CAD build for the part. Positions are in the model's coordinates, mm. A direction names the side the tool comes from. Coordinates: 2 decimals unless noted, no trailing zeros. Write each loop counter-clockwise with the first axis right and the second up, starting at its lowest first coordinate (ties: lowest second). Pieces come first, ordered by that corner, then holes. Notation, with made-up numbers: (79.25, 60.5) - (89.25, 60.5) arc R18 ccw to (89.25, 90.5) - close; hole circle Ø8 at (32, -17.75). An arc over 180 degrees is marked (long way). Answer in a Markdown table with one row per item. Add a question column.
Q1. 3-axis set-ups, long thin cutter, end or side, ignore diameter. For faces 1 (the flat face through (0, 518, 372)), 2 (the flat face through (-25, 50, 321)), 3 (the flat face through (-50, 525, 321)): which of +Z, -Z, +X, -X, +Y, -Y reach the whole face in a straight line?
Q2. Band-saw the part on B-B (y = 481). List the corners of the cut face in (x, z).
Q3. Drill centre lines: line 1 along Z through (x, y) = (-387, 292); line 2 along Y through (x, z) = (-505.5, 617.5); line 3 along Y through (x, z) = (-517.5, 272.5). Where is each one in solid material? Low to high. Write a range as from..to.
Q4. Band-saw the part on C-C (x = -184). List the corners of the cut face in (y, z).
Q5. Band-saw the part on A-A (z = 113). List the corners of the cut face in (x, y).
Q6. Two-plate mould, pull along Y, no slides. Class faces 4 (the flat face through (-516, 550, 320)), 5 (the flat face through (-279, 279, 600)), 6 (the flat face through (-50, 25, 321)): +Y half, -Y half, draft (parallel to the pull), parting line (faces both ways), or undercut.
Q7. Band-saw the part on D-D (x = -510). List the corners of the cut face in (y, z).
Q8. Pin check, flat tips, straight feed: pin 1 (25 mm diameter, centred on y = 17.5, z = 460.5, fed in from +X); pin 2 (25 mm diameter, centred on y = -38.5, z = 151.5, fed in from -X); pin 3 (1.4 mm diameter, centred on x = 1, z = 153.5, fed in from +Y). Stop position of each tip, or through.
```python
from build123d import *

# Parameters (mm, degrees)
F0_W     = 550
F0_H     = 550
F1_DEPTH = 50
F2_W     = 50
F2_H     = 50
F3_DEPTH = 550
F4_W     = 50
F4_H     = 50
F5_DEPTH = 50
F6_W     = 82.6920196414
F6_H     = 273.0440795422
F6_W_2   = 143.6941742897
F6_H_2   = 223.0440795422
F7_DEPTH = 1.8


with BuildPart() as f1:
    # F0 (on Top) → F1 (new body)
    with BuildSketch(Plane.XY):
        with Locations((-275, 275)):
            Rectangle(F0_W, F0_H)
    extrude(amount=F1_DEPTH)

    # F2 (on face) → F3 (join)
    with BuildSketch(Plane.XY.offset(50)):
        with Locations((-525, 525)):
            Rectangle(F2_W, F2_H)
        with Locations((-525, 25)):
            Rectangle(F2_W, F2_H)
        with Locations((-25, 25)):
            Rectangle(F2_W, F2_H)
        with Locations((-25, 525)):
            Rectangle(F2_W, F2_H)
    extrude(amount=F3_DEPTH)

    # F4 (on face) → F5 (join)
    with BuildSketch(Plane.XY.offset(600)):
        with Locations((-525, 525)):
            Rectangle(F4_W, F4_H)
        Polygon((0, 550), (-500, 550), (-500, 500), (-550, 500), (-550, 0), (0, 0), align=None)
    extrude(amount=F5_DEPTH)

    # F6 (on face) → F7 (join)
    with BuildSketch(Plane.YZ):
        with Locations((-41.3460098207, 136.5220397711)):
            Rectangle(F6_W, F6_H)
        Polygon((0, 0), (193.6941742897, 0), (193.6941742897, 50), (50, 50), (50, 273.0440795422), (0, 273.0440795422), align=None)
        with Locations((121.8470871449, 161.5220397711)):
            Rectangle(F6_W_2, F6_H_2)
    extrude(amount=F7_DEPTH)


solid = f1.part
```
Checked values:
| question | item | result |
|---|---|---|
| 1 | face 1 | +Z, +X, +Y |
| 1 | face 2 | -X |
| 1 | face 3 | +Y, -Y |
| 2 | outline | (-550, 0) - (0, 0) - (0, 50) - (-550, 50) - close; (-550, 600) - (0, 600) - (0, 650) - (-550, 650) - close |
| 3 | line 1 | z = 0..50, 600..650 |
| 3 | line 2 | y = 0..550 |
| 3 | line 3 | y = 0..50, 500..550 |
| 4 | outline | (0, 0) - (550, 0) - (550, 50) - (0, 50) - close; (0, 600) - (550, 600) - (550, 650) - (0, 650) - close |
| 5 | outline | (-550, 0) - (-500, 0) - (-500, 50) - (-550, 50) - close; (-550, 500) - (-500, 500) - (-500, 550) - (-550, 550) - close; (-50, 0) - (0, 0) - (0, -82.69) - (1.8, -82.69) - (1.8, 193.69) - (0, 193.69) - (0, 50) - (-50, 50) - close; (-50, 500) - (0, 500) - (0, 550) - (-50, 550) - close |
| 6 | face 4 | +Y half |
| 6 | face 5 | undercut |
| 6 | face 6 | draft |
| 7 | outline | (0, 0) - (550, 0) - (550, 650) - (0, 650) - close; hole (50, 50) - (500, 50) - (500, 600) - (50, 600) - close |
| 8 | pin 1 | stops at x = 0 |
| 8 | pin 2 | stops at x = 0 |
| 8 | pin 3 | stops at y = 193.69 |
